Autodesk Inventor part; units mm, degrees
ref_plane "Work Plane1" through (0, -6.818, 6.8414) normal (0, -1, 0) x (1, 0, 0)
ref_plane "YZ Plane" through (0, 0, 0) normal (1, 0, 0) x (0, 1, 0)
ref_plane "XZ Plane" through (0, 0, 0) normal (0, 1, 0) x (-1, 0, 0)
sketch "Sketch8" plane through (0, 0, 0) normal (1, 0, 0) x (0, 1, 0)
  line L0 (-3.8078, 7.851) -> (3.0591, -12.6251)
  line L1 (-0.2897, -12.6251) -> (-4.6863, 0.485)
  line L2 (3.0591, -12.6251) -> (-0.2897, -12.6251)
  line L3 (-4.6863, 0.485) -> (-6.818, 6.8414)
  line L4 (-3.8078, 7.851) -> (-6.818, 6.8414)
  point P0 (0, 0)
  dimension "d149" = 21.5968
  dimension "d150" = 3.175
  dimension "d151" = 3.3488
extrude "Extrusion6" add sketch "Sketch8" along normal blind 45.72
sketch "Sketch11" plane through (0, 0, 0) normal (-1, 0, 0) x (0, 0, 1)
  line L0 (0.485, -4.6863) -> (-12.6251, -0.2897)
  line L1 (6.8422, -6.8159) -> (6.835, -6.8159)
  line L2 (-12.6251, -0.2897) -> (0.485, -4.6863)
  line L3 (7.851, -3.8078) -> (-12.6251, 3.0591)
  line L4 (13.9082, 14.2533) -> (7.851, -3.808)
  line L5 (7.851, -3.808) -> (-18.639, 5.076)
  line L6 (-18.639, 5.076) -> (-12.5817, 23.1373)
  line L7 (-12.5817, 23.1373) -> (13.9082, 14.2533)
  line L8 (-12.6251, -0.2897) -> (6.8414, -6.818)
  line L9 (6.8414, -6.818) -> (7.851, -3.8078)
  point P0 (0, 0)
  dimension "d73" = 27.94
  dimension "d76" = 0
  dimension "d88" = 19.05
extrude "Extrusion8" add sketch "Sketch11" along normal blind 6.35 contours L3 L5 L6 L7 L4
sketch "Sketch13" plane through (0, -3.8078, 7.851) normal (0, 0.9481042, 0.3179598) x (1, 0, 0)
  line L0 (0, 0) -> (0, 21.5968)
  line L1 (16.51, 18.0408) -> (29.21, 18.0408)
  line L2 (29.21, 18.0408) -> (29.21, 10.4208)
  line L3 (29.21, 10.4208) -> (16.51, 10.4208)
  line L4 (16.51, 10.4208) -> (16.51, 18.0408)
  point P0 (0, 8.6543)
  dimension "d55" = 7.62
  dimension "d56" = 12.7
  dimension "d57" = 16.51
extrude "Extrusion10" cut sketch "Sketch13" against normal blind 25.4
sketch "Sketch15" plane through (0, 0, 0) normal (1, 0, 0) x (0, 0, -1)
  line L0 (6.5678, 21.1205) -> (12.5883, 23.1395)
  line L1 (12.5883, 23.1395) -> (18.6455, 5.0782)
  line L2 (18.6455, 5.0782) -> (12.6251, 3.0591)
  line L3 (12.6251, 3.0591) -> (6.5678, 21.1205)
  dimension "d67" = 6.35
  dimension "d69" = 0
  dimension "d70" = 0
  dimension "d87" = 19.05
extrude "Extrusion11" add sketch "Sketch15" along normal blind 45.72
sketch "Sketch17" plane through (45.72, 0, 0) normal (1, 0, 0) x (0, 0, -1)
  line L0 (-7.851, -3.808) -> (-13.9082, 14.2533)
  line L1 (-7.851, -3.808) -> (-13.9082, 14.2533)
  line L2 (-13.9082, 14.2533) -> (12.5883, 23.1395)
  line L3 (12.5883, 23.1395) -> (18.6456, 5.0782)
  line L4 (18.6456, 5.0782) -> (-7.851, -3.808)
  point P0 (0, 0)
extrude "Extrusion12" add sketch "Sketch17" along normal blind 6.35
sketch "Sketch19" plane through (45.72, 5.0782, -18.6456) normal (0, -0.9481019, -0.3179666) x (1, 0, 0)
  line L0 (0, 6.3501) -> (0, 0.0001)
  line L1 (6.35, 27.947) -> (0, 27.947)
  line L2 (0, 27.947) -> (0, 0.0001)
  line L3 (0, 0.0001) -> (6.35, 0.0001)
  line L4 (6.35, 0.0001) -> (6.35, 27.947)
  line L5 (-45.72, 6.3501) -> (0, 6.3501)
  line L6 (0, 0.0001) -> (0, 0.0001)
  line L7 (0, 0.0001) -> (0, 6.3501)
  line L8 (0, 6.3501) -> (0, 6.3501)
  line L9 (0, 6.3501) -> (0, 0.0001)
  line L10 (-45.72, 0.007) -> (-52.07, 0.007)
  line L11 (-52.07, 0.007) -> (-45.72, 0.007)
  line L12 (-45.72, 0.007) -> (-45.72, 27.947)
  line L13 (-45.72, 27.947) -> (-52.07, 27.947)
  line L14 (-52.07, 27.947) -> (-52.07, 0.007)
  point P0 (-45.72, 19.2926)
extrude "Extrusion13" add sketch "Sketch19" along normal blind 3.175
sketch "Sketch20" plane through (0, 5.0782, -18.6455) normal (0, -0.9481019, -0.3179666) x (1, 0, 0)
  line L0 (45.72, 0) -> (0, 0)
  line L1 (0, 0) -> (0, 6.35)
  line L2 (0, 6.35) -> (45.72, 6.35)
  line L3 (45.72, 6.35) -> (45.72, 0)
  point P0 (0, 19.2926)
extrude "Extrusion14" add sketch "Sketch20" along normal blind 3.175
sketch "Sketch21" plane through (0, 0, 0) normal (1, 0, 0) x (0, 0, -1)
  line L0 (19.6485, 2.0658) -> (13.6346, 0.0489)
  line L1 (13.6346, 0.0489) -> (12.6251, 3.0591)
  line L2 (12.6251, 3.0591) -> (12.6251, -0.2897)
  line L3 (12.6251, -0.2897) -> (-6.8414, -6.818)
  line L4 (-0.485, -4.6863) -> (-0.485, -4.6865)
  line L5 (19.6485, 2.0657) -> (-6.8414, -6.8182)
  line L6 (19.6485, 2.0657) -> (19.6485, 2.0658)
  line L7 (12.6251, 3.0591) -> (13.6346, 0.0489)
  line L8 (12.6251, -0.2897) -> (13.6346, 0.0489)
  line L9 (12.6251, 3.0591) -> (12.6251, -0.2897)
  point P0 (0, 0)
  point P1 (-6.8415, -6.8181)
extrude "Extrusion15" add sketch "Sketch21" along normal blind 45.72
sketch "Sketch22" plane through (16.51, -1.0818, -10.2631) normal (0, 0.9481042, 0.3179598) x (1, 0, 0)
  line L0 (12.7, -7.62) -> (12.7, 0)
  line L1 (12.7, 0) -> (0, 0)
  line L2 (0, 0) -> (12.7, 0)
  line L3 (12.7, 0) -> (12.7, -7.62)
  line L4 (12.7, -7.62) -> (0, -7.62)
  line L5 (0, -7.62) -> (0, 0)
  point P0 (-16.51, -9.3866)
extrude "Extrusion16" cut sketch "Sketch22" against normal blind 45.72
ref_plane "Work Plane1" through (0, -6.818, 6.8414) normal (0, -1, 0) x (1, 0, 0)
sketch "Sketch31" plane through (0, 21.1205, -6.5678) normal (0, -0.3179666, 0.9481019) x (1, 0, 0)
  line L0 (0, -19.05) -> (45.72, -19.05)
  line L1 (8.11, -16.025) -> (37.61, -16.025)
  line L2 (37.61, -16.025) -> (37.61, -13.275)
  line L3 (37.61, -13.275) -> (41.36, -13.275)
  arc A0 (41.36, -13.275) -> (41.36, -5.775) centre (41.36, -9.525) ccw
  line L4 (41.36, -5.775) -> (37.61, -5.775)
  line L5 (37.61, -5.775) -> (37.61, -3.025)
  line L6 (37.61, -3.025) -> (8.11, -3.025)
  line L7 (8.11, -3.025) -> (8.11, -5.775)
  line L8 (8.11, -5.775) -> (4.36, -5.775)
  arc A1 (4.36, -5.775) -> (4.36, -13.275) centre (4.36, -9.525) ccw
  line L9 (4.36, -13.275) -> (8.11, -13.275)
  line L10 (8.11, -13.275) -> (8.11, -16.025)
  circle A2 centre (41.36, -9.525) radius 1.6
  circle A3 centre (4.36, -9.525) radius 1.6
  line L11 (22.86, -3.025) -> (22.86, -16.025)
  line L12 (0, 0) -> (45.72, 0)
  line L13 (22.86, 0) -> (22.86, -19.05)
  line L14 (4.36, -9.525) -> (41.36, -9.525)
  line L15 (0, -22.225) -> (0, 0)
  line L16 (45.72, -19.05) -> (45.72, 0)
  line L17 (0, -9.525) -> (45.72, -9.525)
  point P0 (0, -17.936)
  point P1 (22.86, -9.525)
  point P2 (22.86, -9.525)
  dimension "d132" = 9.525
extrude "Extrusion24" cut sketch "Sketch31" against normal through all contours L17 L14 A3 | A3 L14 L17 | L14 L17 A2 | A2 L17 L14
sketch "Sketch32" plane through (52.07, 0, 0) normal (1, 0, 0) x (0, 0, -1)
  line L0 (19.6551, 2.0679) -> (-6.8414, -6.8182)
  line L1 (-6.8414, -6.8182) -> (-6.8414, -25.8682)
  line L2 (-6.8414, -25.8682) -> (19.6551, -25.8682)
  line L3 (19.6551, -25.8682) -> (19.6551, 2.0679)
  point P0 (0, 0)
  dimension "d139" = 19.05
extrude "Extrusion25" add sketch "Sketch32" against normal up to surface (6.35 mm away)
sketch "Sketch33" plane through (-6.35, 0, 0) normal (-1, 0, 0) x (0, 0, 1)
  line L0 (6.8414, -25.8682) -> (6.8414, -6.8182)
  line L1 (-19.6551, -25.8682) -> (6.8414, -25.8682)
  line L2 (-19.6551, 2.0679) -> (-19.6551, -25.8682)
  line L3 (13.9082, 14.2533) -> (6.8414, -6.8182)
  line L4 (-19.6551, 2.0679) -> (6.8414, -6.8182)
  point P0 (0, 0)
extrude "Extrusion26" add sketch "Sketch33" against normal up to surface (6.35 mm away)
sketch "Sketch34" plane through (52.07, 0, 0) normal (1, 0, 0) x (0, 0, -1)
  line L0 (-6.8414, -25.8682) -> (-6.8414, -6.8182)
  line L1 (19.6551, -25.8682) -> (-6.8414, -25.8682)
  circle A0 centre (6.4047, -16.5549) radius 3.302
  point P0 (0, 0)
  dimension "d144" = 6.604
  dimension "d145" = 9.3133
  dimension "d146" = 13.2461
extrude "Extrusion27" cut sketch "Sketch34" against normal up to surface (58.42 mm away)
equation "\"d57\" = d58"
properties part number "Lidar Sensor Case v3"
Geometry check sheet. Reference: the model listing, model coordinates, mm. A direction names the side the tool comes from. Give positions to 0.01 mm unless a question says otherwise; leave off trailing zeros. Write each loop counter-clockwise with the first axis right and the second up, starting at its lowest first coordinate (ties: lowest second). Pieces come first, ordered by that corner, then holes. Notation, with made-up numbers: (-6.5, 42.5) - (8.5, 42.5) arc R18 cw to (8.5, 73.5) - close; hole circle Ø11 at (-13, 20). An arc over 180 degrees is marked (long way). Put each result on its own line as item: value.
1. Thickness scan on line 1 (X direction, y = 3.5, z = -4); line 2 (X direction, y = 13, z = -11.5); line 3 (Y direction, x = 48, z = -12.5). Record the ranges inside material, lowest first.
Ans:
line 1: x = -6.35 to 0, 45.72 to 52.07
line 2: x = -6.35 to 2.78, 5.94 to 39.78, 42.94 to 52.07
line 3: y = -25.87 to 23.11
2. Sectioned sample at B-B, the plane z = 11. Enter the section's corners in (x, y), plus the area to 3 significant figures.
Ans:
outline: (-6.35, 5.58) - (0, 5.58) - (0, 15.23) - (-6.35, 15.23) - close; (45.72, 5.58) - (52.07, 5.58) - (52.07, 15.23) - (45.72, 15.23) - close
area: 123 mm²
3. Go/stop test with flat-tipped pins: pin 1 (5 mm diameter, centred on x = 47.5, y = -14, fed in from +Z); pin 2 (2 mm diameter, centred on x = 9.5, z = -14, fed in from -Y); pin 3 (1.5 mm diameter, centred on x = 34.5, y = -6, fed in from +Z). Record where each tip stops, or that it passes through.
Ans:
pin 1: stops at z = 6.84
pin 2: stops at y = -0.16
pin 3: stops at z = 7.37
4. Sectioned sample at A-A, the plane y = -9.5. Enter the section's corners in (x, z).
Ans:
outline: (-6.35, -19.66) - (0, -19.66) - (0, 6.84) - (-6.35, 6.84) - close; (45.72, -19.66) - (52.07, -19.66) - (52.07, 6.84) - (45.72, 6.84) - close
5. Draft check along Z on faces 1 (the flat face through (-3, -16, 6.841)), 2 (the flat face through (16.51, -1, -6)), 3 (the flat face through (45.72, 9, 1)). Enter one of: +Z half, -Z half, draft (parallel to the pull), parting line (faces both ways), or undercut.
Ans:
face 1: +Z half
face 2: undercut
face 3: draft
6. Sectioned sample at C-C, the plane y = -18. Enter the section's corners in (x, z).
Ans:
outline: (-6.35, -19.66) - (0, -19.66) - (0, -9.37) - (-6.35, -9.37) - close; (-6.35, -3.44) - (0, -3.44) - (0, 6.84) - (-6.35, 6.84) - close; (45.72, -19.66) - (52.07, -19.66) - (52.07, -9.37) - (45.72, -9.37) - close; (45.72, -3.44) - (52.07, -3.44) - (52.07, 6.84) - (45.72, 6.84) - close
7. Set-up check for faces 4 (the flat face through (0, -12, -7)), 5 (the flat face through (22.771, 0.444, -9.751)), 6 (the flat face through (49, -25.868, -6)), 7 (the flat face through (22.54, -1.185, 0.031)), 8 (the flat face through (49, -16, 6.841)): record each of +Z, -Z, +X, -X, +Y, -Y from which the full face is reachable in a straight line by a thin tool's end or side.
Ans:
face 4: -Z, -Y
face 5: -Y
face 6: +Z, -Z, +X, -X, -Y
face 7: +Z
face 8: +Z, +X, -X, -Y
8. Sectioned sample at D-D, the plane x = 17.5. Enter the section's corners in (y, z) (1 decimal).
Ans:
outline: (-6.8, 6.8) - (-4.7, 0.5) - (-3.5, -3) - (-0.5, -2) - (-3.8, 7.9) - close; (-1.1, -10.3) - (-0.3, -12.6) - (0, -13.6) - (2.1, -19.7) - (5.1, -18.6) - (23.1, -12.6) - (21.1, -6.6) - (3.1, -12.6) - (1.9, -9.3) - close
